```python
from build123d import *

# Parameters (mm, degrees)
EXTRUDE_1_DEPTH      = 3
SKETCH_2_W           = 3
SKETCH_2_H           = 35
CUT_EXTRUDE_1_DEPTH  = 3
CUT_EXTRUDE_2_DEPTH  = 3
SKETCH_4_W           = 3
SKETCH_4_H           = 10
CUT_EXTRUDE_3_DEPTH  = 3
SKETCH_5_W           = 15
SKETCH_5_H           = 3
CUT_EXTRUDE_4_DEPTH  = 3
SKETCH_6_W           = 324.73
SKETCH_6_H           = 3
EXTRUDE_2_DEPTH      = 6
SKETCH_8_W           = 3
SKETCH_8_H           = 3
SKETCH_9_W           = 3
SKETCH_9_H           = 3
SKETCH_7_R           = 1.5
CUT_EXTRUDE_6_DEPTH  = 3
FILLET_1_R           = 3
SKETCH_14_R          = 1.5
CUT_EXTRUDE_9_DEPTH  = 3
SKETCH_15_R          = 1.5
CUT_EXTRUDE_10_DEPTH = 3
SKETCH_16_W          = 3
SKETCH_16_H          = 3
SKETCH_17_W          = 3
SKETCH_17_H          = 3
SKETCH_18_R          = 1.5
CUT_EXTRUDE_11_DEPTH = 3
FILLET_2_R           = 3
CHAMFER_1_SIZE2      = 3.464101615
CHAMFER_1_SIZE       = 6
SKETCH_19_R          = 36
CUT_EXTRUDE_12_DEPTH = 3
SKETCH_24_W          = 20
SKETCH_24_H          = 3
SKETCH_24_W_2        = 60
EXTRUDE_3_DEPTH      = 3
CUT_EXTRUDE_13_DEPTH = 3
FILLET_3_R           = 1
SKETCH_26_W          = 3
SKETCH_26_H          = 20
CUT_EXTRUDE_14_DEPTH = 3


with BuildPart() as part:
    # Эскиз1 → Бобышка-Вытянуть1 (new body)
    with BuildSketch(Plane.XY):
        Polygon((-42.146569651, 73), (0, 0), (-366.876569651, 0), (-366.876569651, 73), align=None)
    extrude(amount=EXTRUDE_1_DEPTH)

    # Эскиз2 → Вырез-Вытянуть1 (cut)
    with BuildSketch(Plane.XY.offset(3)):
        with Locations((-365.376569651, 35)):
            Rectangle(SKETCH_2_W, SKETCH_2_H)
    extrude(amount=-CUT_EXTRUDE_1_DEPTH, mode=Mode.SUBTRACT)

    # Эскиз3 → Вырез-Вытянуть2 (cut)
    with BuildSketch(Plane.XY.offset(3)):
        Polygon((-33.287386441, 51.655444566), (-30.689310229, 53.155444566), (-13.189310229, 22.844555434), (-15.787386441, 21.344555434), align=None)
    extrude(amount=-CUT_EXTRUDE_2_DEPTH, mode=Mode.SUBTRACT)

    # Эскиз4 → Вырез-Вытянуть3 (cut)
    with BuildSketch(Plane.XY.offset(3)):
        with Locations((-240.376569651, 35)):
            Rectangle(SKETCH_4_W, SKETCH_4_H)
        with Locations((-156.376569651, 35)):
            Rectangle(SKETCH_4_W, SKETCH_4_H)
    extrude(amount=-CUT_EXTRUDE_3_DEPTH, mode=Mode.SUBTRACT)

    # Эскиз5 → Вырез-Вытянуть4 (cut)
    with BuildSketch(Plane.XY.offset(3)):
        with Locations((-336.376569651, 35)):
            Rectangle(SKETCH_5_W, SKETCH_5_H)
        with Locations((-52.036569651, 35)):
            Rectangle(SKETCH_5_W, SKETCH_5_H)
    extrude(amount=-CUT_EXTRUDE_4_DEPTH, mode=Mode.SUBTRACT)

    # Эскиз6 → Бобышка-Вытянуть2 (add)
    with BuildSketch(Plane(origin=(0, 73, 0), x_dir=(1, 0, 0), z_dir=(0, 1, 0))):
        with Locations((-204.511569651, -1.5)):
            Rectangle(SKETCH_6_W, SKETCH_6_H)
    extrude(amount=EXTRUDE_2_DEPTH)

    # Эскиз8 → Повернуть1 (revolve)
    with BuildSketch(Plane.ZY.offset(366.876569651)):
        with Locations((1.5, 7.25)):
            Rectangle(SKETCH_8_W, SKETCH_8_H)
    revolve(axis=Axis((-366.876569651, 8.75, 0), (0, 0, 1)))

    # Эскиз9 → Повернуть2 (revolve)
    with BuildSketch(Plane.ZY.offset(366.876569651)):
        with Locations((1.5, 59.75)):
            Rectangle(SKETCH_9_W, SKETCH_9_H)
    revolve(axis=Axis((-366.876569651, 61.25, 0), (0, 0, 1)))

    # Эскиз7 → Вырез-Вытянуть6 (cut)
    with BuildSketch(Plane.XY.offset(3)):
        with Locations((-365.376569651, 8.75)):
            Circle(SKETCH_7_R)
        with Locations(Location((-365.376569651, 61.25, 0), (0, 0, 180))):
            Circle(SKETCH_7_R)
    extrude(amount=-CUT_EXTRUDE_6_DEPTH, mode=Mode.SUBTRACT)

    # Скругление1
    fillet_1_edges = [part.edges().sort_by_distance(p)[0] for p in [
        (-366.876569651, 5.75, 1.5),
        (-366.876569651, 11.75, 1.5),
        (-366.876569651, 58.25, 1.5),
        (-366.876569651, 64.25, 1.5),
    ]]
    fillet(fillet_1_edges, radius=FILLET_1_R)

    # Эскиз14 → Вырез-Вытянуть9 (cut)
    with BuildSketch(Plane.XY.offset(3)):
        with Locations((-156.376569651, 43.5)):
            Circle(SKETCH_14_R)
        with Locations((-156.376569651, 26.5)):
            Circle(SKETCH_14_R)
        with Locations((-240.376569651, 26.5)):
            Circle(SKETCH_14_R)
        with Locations((-240.376569651, 43.5)):
            Circle(SKETCH_14_R)
    extrude(amount=-CUT_EXTRUDE_9_DEPTH, mode=Mode.SUBTRACT)

    # Эскиз15 → Вырез-Вытянуть10 (cut)
    with BuildSketch(Plane.XY.offset(3)):
        with Locations((-324.376569651, 35)):
            Circle(SKETCH_15_R)
        with Locations((-348.376569651, 35)):
            Circle(SKETCH_15_R)
        with Locations((-64.036569651, 35)):
            Circle(SKETCH_15_R)
        with Locations((-40.036569651, 35)):
            Circle(SKETCH_15_R)
    extrude(amount=-CUT_EXTRUDE_10_DEPTH, mode=Mode.SUBTRACT)

    # Эскиз16 → Повернуть3 (revolve)
    with BuildSketch(Plane(origin=(0, 0, 0), x_dir=(0, 0, -1), z_dir=(0.8660254037844265, 0.5000000000000212, 0))):
        with Locations((-1.5, 12.558620458)):
            Rectangle(SKETCH_16_W, SKETCH_16_H)
    revolve(axis=Axis((-7.029310229, 12.175122459, 3), (0, 0, -1)))

    # Эскиз17 → Повернуть4 (revolve)
    with BuildSketch(Plane(origin=(0, 0, 0), x_dir=(0, 0, -1), z_dir=(0.8660254037844265, 0.5000000000000212, 0))):
        with Locations((-1.5, 75.198620458)):
            Rectangle(SKETCH_17_W, SKETCH_17_H)
    revolve(axis=Axis((-36.849310229, 63.824877541, 3), (0, 0, -1)))

    # Эскиз18 → Вырез-Вытянуть11 (cut)
    with BuildSketch(Plane.XY.offset(3)):
        with Locations((-38.149990748, 63.077722283)):
            Circle(SKETCH_18_R)
        with Locations((-8.326705922, 11.422277717)):
            Circle(SKETCH_18_R)
    extrude(amount=-CUT_EXTRUDE_11_DEPTH, mode=Mode.SUBTRACT)

    # Скругление2
    fillet_2_edges = [part.edges().sort_by_distance(p)[0] for p in [
        (-5.529310229, 9.577046248, 1.5),
        (-8.529310229, 14.773198671, 1.5),
        (-35.349310229, 61.226801329, 1.5),
        (-38.349310229, 66.422953752, 1.5),
    ]]
    fillet(fillet_2_edges, radius=FILLET_2_R)

    # Фаска1
    chamfer_1_edges = [part.edges().sort_by_distance(p)[0] for p in [
        (-42.146569651, 79, 1.5),
    ]]
    chamfer_1_side = [part.faces().sort_by_distance(p)[0] for p in [
        (-42.146569651, 78.930717968, 1.5),
    ]]
    chamfer(chamfer_1_edges, length=CHAMFER_1_SIZE - 0.0001, length2=CHAMFER_1_SIZE2 - 0.0001, reference=chamfer_1_side[0])  # a hair under: the kernel refuses the full size

    # Эскиз19 → Вырез-Вытянуть12 (cut)
    with BuildSketch(Plane.XY.offset(3)):
        with Locations((-279.876569651, 25)):
            Circle(SKETCH_19_R)
        with Locations((-113.876569651, 25)):
            Circle(SKETCH_19_R)
    extrude(amount=-CUT_EXTRUDE_12_DEPTH, mode=Mode.SUBTRACT)

    # Эскиз24 → Бобышка-Вытянуть3 (add)
    with BuildSketch(Plane(origin=(0, 79, 0), x_dir=(1, 0, 0), z_dir=(0, 1, 0))):
        with Locations((-66.876569651, -1.5)):
            Rectangle(SKETCH_24_W, SKETCH_24_H)
        with Locations((-136.876569651, -1.5)):
            Rectangle(SKETCH_24_W_2, SKETCH_24_H)
        with Locations((-286.876569651, -1.5)):
            Rectangle(SKETCH_24_W_2, SKETCH_24_H)
    extrude(amount=EXTRUDE_3_DEPTH)

    # Эскиз25 → Вырез-Вытянуть13 (cut)
    with BuildSketch(Plane.XY.offset(3)):
        Polygon((-348.376569651, 79), (-348.376569651, 73), (-349.626569651, 73), (-349.626569651, 70.5), (-348.376569651, 70.5), (-348.376569651, 64.5), (-345.376569651, 64.5), (-345.376569651, 70.5), (-344.126569651, 70.5), (-344.126569651, 73), (-345.376569651, 73), (-345.376569651, 79), align=None)
        Polygon((-218.376569651, 79), (-218.376569651, 73), (-219.626569651, 73), (-219.626569651, 70.5), (-218.376569651, 70.5), (-218.376569651, 64.5), (-215.376569651, 64.5), (-215.376569651, 70.5), (-214.126569651, 70.5), (-214.126569651, 73), (-215.376569651, 73), (-215.376569651, 79), align=None)
        Polygon((-83.376569651, 79), (-83.376569651, 73), (-84.626569651, 73), (-84.626569651, 70.5), (-83.376569651, 70.5), (-83.376569651, 64.5), (-80.376569651, 64.5), (-80.376569651, 70.5), (-79.126569651, 70.5), (-79.126569651, 73), (-80.376569651, 73), (-80.376569651, 79), align=None)
    extrude(amount=-CUT_EXTRUDE_13_DEPTH, mode=Mode.SUBTRACT)

    # Скругление3
    fillet_3_edges = [part.edges().sort_by_distance(p)[0] for p in [
        (0, 0, 1.5),
    ]]
    fillet(fillet_3_edges, radius=FILLET_3_R)

    # Эскиз26 → Вырез-Вытянуть14 (cut)
    with BuildSketch(Plane.XY.offset(3)):
        with Locations((-59.376569651, 50)):
            Rectangle(SKETCH_26_W, SKETCH_26_H)
    extrude(amount=-CUT_EXTRUDE_14_DEPTH, mode=Mode.SUBTRACT)


solid = part.part
```
Work out the finished part from the listing and answer in its coordinate system (mm). Give positions to 0.01 mm unless a question says otherwise; leave off trailing zeros. Write each loop counter-clockwise with the first axis right and the second up, starting at its lowest first coordinate (ties: lowest second). Pieces come first, ordered by that corner, then holes. Notation, with made-up numbers: (-29, 49) -> (-16, 49) arc R31 cw to (-16, 87) -> close; hole circle Ø1 at (71, 88.25). An arc over 180 degrees is marked (long way). Write item = value, one per line.
Q1. For a pull along X with two mould halves and no side action, classify faces 1 (the flat face through (-188, 40, 0)), 2 (the cylindrical face through (-112.7, 60.98, 1.52)), 3 (the cylindrical face through (-278.7, 60.98, 1.52)) as pulls with the +X half, pulls with the -X half, needs draft (parallel to the pull), parting line crosses it, or undercut.
Computed values:
face_1 = needs draft
face_2 = undercut
face_3 = undercut
Q2. Section A-A on x = -53 is taken. Determine the outline of the cut face in (y, z).
Computed values:
outline = (0, 0) -> (33.5, 0) -> (33.5, 3) -> (0, 3) -> close; (36.5, 0) -> (79, 0) -> (79, 3) -> (36.5, 3) -> close
Q3. Flat-ended cylindrical pins translate along their axes: pin 1 Ø0.9 at (y, z) = (75, 2) entering from +X; pin 2 Ø0.9 at (y, z) = (80, 2) entering from +X; pin 3 Ø1.5 at (y, z) = (68, 1) entering from -X. Find the tip coordinate at first contact, or state that the pin passes through.
Computed values:
pin_1 = -43.04
pin_2 = -56.88
pin_3 = -366.88
Q4. Section C-C on x = -113.5 is taken. Determine the outline of the cut face in (y, z), and give its area (3 significant figures).
Computed values:
outline = (61, 0) -> (82, 0) -> (82, 3) -> (61, 3) -> close
area = 63.0 mm^2
Q5. Consider line 1 along X through (y, z) = (48, 1.8); line 2 along X through (y, z) = (65, 2.4); line 3 along Y through (x, z) = (-334, 1.2). Determine where each line is inside the solid, lowest interval first.
Computed values:
line_1 = -363.88 to -307.57, -252.18 to -141.57, -86.18 to -60.88, -57.88 to -31.18
line_2 = -367.25 to -348.38, -345.38 to -218.38, -215.38 to -83.38, -80.38 to -34.09
line_3 = 0 to 33.5, 36.5 to 79
Q6. Section B-B on z = 1.4 is taken. State how many separate pieces and enclosed holes the cut face has, and give its area (3 significant figures).
Computed values:
separate_pieces = 1
enclosed_holes = 17
area = 19,700 mm^2
